Design review of the part built by this model. Coordinates are the model's own, in mm. A direction names the side the tool comes from. Coordinates: 2 decimals unless noted, no trailing zeros. Loops run counter-clockwise (first coordinate to the right, second up) from the corner with the lowest first, then second, coordinate; pieces in that order, holes last. Notation, with made-up numbers: (-35, 18.5) - (20, 18.5) arc R14 cw to (20, 40.5) - close; hole circle Ø5 at (81, 22.25). An arc over 180 degrees is marked (long way). Answer in a Markdown table with one row per item. Add a question column.
(1) For faces 3 (the face through (15, -1, -9)), 4 (the face through (25, 2, -29)), 5 (the face through (11.05, -9.56, -22.65)), list the 3-axis set-ups (+Z, -Z, +X, -X, +Y, -Y) from which the entire face can be reached by the end or side of a thin tool; tool diameter is ignored.
(2) We need section D-D, the plane y = -3. Write out the cut boundary in (x, z), plus the area to 3 significant figures.
(3) The part is to be moulded in two halves that separate along X. For faces 1 (the face through (16.84, 14.94, -19.72)), 2 (the face through (14.79, 12.76, -26.1)), say which applies: released by +X, released by -X, zero draft, split by the parting line, or undercut.
(4) We need section C-C, the plane z = 26. Write out the cut boundary in (x, y), plus the area to 3 significant figures.
(5) We need section A-A, the plane z = 7. Write out the cut boundary in (x, y), plus the area to 3 significant figures.
(6) Clearance check with flat-ended pins moving along their axes: pin 1 (1.7 mm diameter, centred on x = 17, z = -3, fed in from -Y); pin 2 (2 mm diameter, centred on x = 12.5, z = 21.5, fed in from -Y); pin 3 (5 mm diameter, centred on x = 9, y = -8, fed in from -Z). State where each tip first meets the part, or that it passes through.
(7) To check wall thickness, follow L1, parallel to Z at x = 12.5, y = 21; L2, parallel to Y at x = 24, z = 24; L3, parallel to X at y = 22, z = -8.5. State the ranges of each line that lie inside material, in increasing order. Write a range as [from, to].
(8) We need section B-B, the plane y = 21. Write out the cut boundary in (x, z), plus the area to 3 significant figures.
from build123d import *

# Parameters (mm, degrees)
SKETCH_1_R               = 30
EXTRUDE_1_DEPTH          = 30
CUT_EXTRUDE_1_DEPTH      = 31
CUT_EXTRUDE_2_DEPTH      = 31
CUT_EXTRUDE_3_DEPTH      = 9
PATTERN_CIRCULAR_2_COUNT = 12


with BuildPart() as part:
    # Sketch 1 → Extrude 1 (new body)
    with BuildSketch(Plane(origin=(0, 0, 0), x_dir=(0, 0, -1), z_dir=(1, 0, 0))):
        Circle(SKETCH_1_R)
    extrude(amount=EXTRUDE_1_DEPTH)

    # Sketch 2 → Cut-Extrude 1 (cut, through all)
    with BuildSketch(Plane(origin=(0, 0, 0), x_dir=(0, 0, -1), z_dir=(1, 0, 0))):
        Polygon((0, 30), (2, 30), (2, 28), (-2, 28), (-2, 30), align=None)
    cut_extrude_1 = extrude(amount=CUT_EXTRUDE_1_DEPTH, mode=Mode.SUBTRACT)

    # Sketch 3 → Cut-Extrude 2 (cut, through all)
    with BuildSketch(Plane(origin=(0, 0, 0), x_dir=(0, 0, -1), z_dir=(1, 0, 0))):
        with BuildLine():
            Line((4.898979486, -0.999999998), (12.500084161, -0.999999998))
            Line((12.500084161, -0.999999998), (12.5, 1))
            Line((12.5, 1), (4.898979486, 1))
            ThreePointArc((4.898979486, 1), (0, 5), (-4.898979486, 1))
            Line((-4.898979486, 1), (-12.5, 1))
            Line((-12.5, 1), (-12.499915839, -0.999999998))
            Line((-12.499915839, -0.999999998), (-4.898979486, -0.999999998))
            ThreePointArc((-4.898979486, -0.999999998), (0, -5), (4.898979486, -0.999999998))
        make_face()
    extrude(amount=CUT_EXTRUDE_2_DEPTH, mode=Mode.SUBTRACT)

    # Sketch 4 → Cut-Extrude 3 (cut, symmetric)
    with BuildSketch(Plane(origin=(0, 28, 0), x_dir=(1, 0, 0), z_dir=(0, 1, 0))):
        Polygon((14.249202979, -2), (10.006562292, -2), (12.127882636, -4.121320344), align=None)
        Polygon((15.763921605, -2), (20.006562292, -2), (17.885241949, -4.121320344), align=None)
    cut_extrude_3 = extrude(amount=CUT_EXTRUDE_3_DEPTH, both=True, mode=Mode.SUBTRACT)

    # Pattern Circular 2: Cut-Extrude 1, Cut-Extrude 3 ×12 about axis
    pattern_circular_2_axis = Axis((0, 0, 0), (1, 0, 0))
    for i in range(1, PATTERN_CIRCULAR_2_COUNT):
        add(cut_extrude_1.rotate(pattern_circular_2_axis, i * 360 / PATTERN_CIRCULAR_2_COUNT), mode=Mode.SUBTRACT)
        add(cut_extrude_3.rotate(pattern_circular_2_axis, i * 360 / PATTERN_CIRCULAR_2_COUNT), mode=Mode.SUBTRACT)


solid = part.part
Responses:
| question | item | result |
|---|---|---|
| 1 | face 3 | +X, -X |
| 1 | face 4 | -Z, +X, -X |
| 1 | face 5 | none |
| 2 | outline | (0, -29.85) - (30, -29.85) - (30, -4) - (0, -4) - close; (0, 4) - (30, 4) - (30, 29.85) - (19.01, 29.85) - (19.01, 19) - (16.76, 19) - (16.76, 29.85) - (13.25, 29.85) - (13.25, 19) - (11.01, 19) - (11.01, 29.85) - (0, 29.85) - close |
| 2 | area | 1,500 mm2 |
| 3 | face 1 | undercut |
| 3 | face 2 | zero draft |
| 4 | outline | (0, -12.7) - (30, -12.7) - (30, 12.7) - (20.01, 12.7) - (17.89, 10.25) - (15.76, 12.7) - (14.25, 12.7) - (12.13, 10.25) - (10.01, 12.7) - (0, 12.7) - close; hole (10.01, -2) - (12.13, -4.12) - (14.25, -2) - close; hole (15.76, -2) - (17.89, -4.12) - (20.01, -2) - close |
| 4 | area | 743 mm2 |
| 5 | outline | (0, -29.17) - (30, -29.17) - (30, -1) - (0, -1) - close; (0, 1) - (30, 1) - (30, 29.17) - (0, 29.17) - close; hole (10.89, -17.9) - (12.13, -20.37) - (13.36, -17.9) - close; hole (16.65, -17.9) - (17.89, -20.37) - (19.12, -17.9) - close |
| 5 | area | 1,680 mm2 |
| 6 | pin 1 | stops at y = -29.89 |
| 6 | pin 2 | stops at y = -21.9 |
| 6 | pin 3 | stops at z = -29.49 |
| 7 | L1 | z = [-21.42, -9.81], [-7.8, 2], [3.75, 14.43], [16.45, 21.42] |
| 7 | L2 | y = [-18, -16.17], [-14.43, 14.43], [16.17, 18] |
| 7 | L3 | x = [0, 11.65], [12.61, 17.4], [18.37, 30] |
| 8 | outline | (0, -21.42) - (30, -21.42) - (30, 21.42) - (0, 21.42) - close; hole (10.01, -9.81) - (14.25, -9.81) - (12.13, -7.37) - close; hole (10.01, 2) - (14.25, 2) - (12.13, 4.12) - close; hole (10.01, 14.43) - (14.25, 14.43) - (12.13, 16.88) - close; hole (15.76, -9.81) - (20.01, -9.81) - (17.89, -7.37) - close; hole (15.76, 2) - (20.01, 2) - (17.89, 4.12) - close; hole (15.76, 14.43) - (20.01, 14.43) - (17.89, 16.88) - close |
| 8 | area | 1,260 mm2 |
